```python
from build123d import *

# Parameters (mm, degrees)
SKETCH_2_W          = 110
SKETCH_2_H          = 80
EXTRUDE_1_DEPTH     = 4
EXTRUDE_1_2_DEPTH   = 76
EXTRUDE_2_DEPTH     = 2
CUT_EXTRUDE_1_DEPTH = 90.5
SKETCH_6_R          = 5.5
CUT_EXTRUDE_2_DEPTH = 5
FILLET_1_R          = 10
CUT_EXTRUDE_3_REACH = 61


with BuildPart() as part:
    # Эскиз2 → Extrude 1 (new body)
    with BuildSketch(Plane(origin=(0, 0, 0), x_dir=(1, 0, 0), z_dir=(0, 1, 0))):
        Rectangle(SKETCH_2_W, SKETCH_2_H)
    extrude(amount=EXTRUDE_1_DEPTH)

    # Эскиз3 → Extrude 1 2 (add)
    with BuildSketch(Plane(origin=(0, 4, 0), x_dir=(1, 0, 0), z_dir=(0, 1, 0))):
        with BuildLine():
            Line((-30.5, -15), (-30.5, 14))
            ThreePointArc((-30.5, 14), (-30.207106781, 14.707106781), (-29.5, 15))
            Line((-29.5, 15), (29.5, 15))
            ThreePointArc((29.5, 15), (30.207106781, 14.707106781), (30.5, 14))
            Line((30.5, 14), (30.5, -15))
            Line((30.5, -15), (34.5, -15))
            Line((34.5, -15), (34.5, 14))
            ThreePointArc((34.5, 14), (33.035533906, 17.535533906), (29.5, 19))
            Line((29.5, 19), (-29.5, 19))
            ThreePointArc((-29.5, 19), (-33.035533906, 17.535533906), (-34.5, 14))
            Line((-34.5, 14), (-34.5, -15))
            Line((-34.5, -15), (-30.5, -15))
        make_face()
    extrude(amount=EXTRUDE_1_2_DEPTH)

    # Эскиз4 → Бобышка-Вытянуть2 (add, symmetric)
    with BuildSketch(Plane(origin=(0, 0, 0), x_dir=(0, 0, -1), z_dir=(1, 0, 0))):
        Polygon((19, 31.712812921), (35, 4), (19, 4), align=None)
    extrude(amount=EXTRUDE_2_DEPTH, both=True)

    # Эскиз5 → Вырез-Вытянуть1 (cut, through all)
    with BuildSketch(Plane(origin=(34.5, 0, 0), x_dir=(0, 0, -1), z_dir=(1, 0, 0))):
        with BuildLine():
            Line((5, 68), (5, 56))
            ThreePointArc((5, 56), (0, 51), (-5, 56))
            Line((-5, 56), (-5, 68))
            ThreePointArc((-5, 68), (0, 73), (5, 68))
        make_face()
        with BuildLine():
            Line((5, 28), (5, 16))
            ThreePointArc((5, 16), (0, 11), (-5, 16))
            Line((-5, 16), (-5, 28))
            ThreePointArc((-5, 28), (0, 33), (5, 28))
        make_face()
    extrude(amount=-CUT_EXTRUDE_1_DEPTH, mode=Mode.SUBTRACT)

    # Эскиз6 → Вырез-Вытянуть2 (cut, through all)
    with BuildSketch(Plane(origin=(0, 4, 0), x_dir=(1, 0, 0), z_dir=(0, 1, 0))):
        with Locations(Location((-43, 28, 0), (0, 0, 270))):  # turned: the seam where the file's is
            Circle(SKETCH_6_R)
        with Locations(Location((-43, -28, 0), (0, 0, 270))):  # turned: the seam where the file's is
            Circle(SKETCH_6_R)
        with Locations(Location((43, 28, 0), (0, 0, 270))):  # turned: the seam where the file's is
            Circle(SKETCH_6_R)
        with Locations(Location((43, -28, 0), (0, 0, 270))):  # turned: the seam where the file's is
            Circle(SKETCH_6_R)
    extrude(amount=-CUT_EXTRUDE_2_DEPTH, mode=Mode.SUBTRACT)

    # Скругление1
    fillet_1_edges = [part.edges().sort_by_distance(p)[0] for p in [
        (55, 2, 40),
        (-55, 2, 40),
        (-55, 2, -40),
        (55, 2, -40),
    ]]
    fillet(fillet_1_edges, radius=FILLET_1_R)

    # Эскиз8 → Вырез-Вытянуть3 (cut, up to next)
    with BuildSketch(Plane(origin=(0, 0, -19), x_dir=(-1, 0, 0), z_dir=(0, 0, -1)), mode=Mode.PRIVATE) as cut_extrude_3_sk1:
        with BuildLine():
            Line((-10, 68), (-10, 56))
            ThreePointArc((-10, 56), (-15, 51), (-20, 56))
            Line((-20, 56), (-20, 68))
            ThreePointArc((-20, 68), (-15, 73), (-10, 68))
        make_face()
    cut_extrude_3_tool1 = extrude(cut_extrude_3_sk1.sketch, amount=-CUT_EXTRUDE_3_REACH, mode=Mode.PRIVATE) & part.part
    add(cut_extrude_3_tool1.solids().sort_by_distance((15, 62, -19))[0], mode=Mode.SUBTRACT)
    # Эскиз8 → Вырез-Вытянуть3 (cut, up to next)
    with BuildSketch(Plane(origin=(0, 0, -19), x_dir=(-1, 0, 0), z_dir=(0, 0, -1)), mode=Mode.PRIVATE) as cut_extrude_3_sk2:
        with BuildLine():
            Line((-10, 28), (-10, 16))
            ThreePointArc((-10, 16), (-15, 11), (-20, 16))
            Line((-20, 16), (-20, 28))
            ThreePointArc((-20, 28), (-15, 33), (-10, 28))
        make_face()
    cut_extrude_3_tool2 = extrude(cut_extrude_3_sk2.sketch, amount=-CUT_EXTRUDE_3_REACH, mode=Mode.PRIVATE) & part.part
    add(cut_extrude_3_tool2.solids().sort_by_distance((15, 22, -19))[0], mode=Mode.SUBTRACT)
    # Эскиз8 → Вырез-Вытянуть3 (cut, up to next)
    with BuildSketch(Plane(origin=(0, 0, -19), x_dir=(-1, 0, 0), z_dir=(0, 0, -1)), mode=Mode.PRIVATE) as cut_extrude_3_sk3:
        with BuildLine():
            Line((10, 68), (10, 56))
            ThreePointArc((10, 56), (15, 51), (20, 56))
            Line((20, 56), (20, 68))
            ThreePointArc((20, 68), (15, 73), (10, 68))
        make_face()
    cut_extrude_3_tool3 = extrude(cut_extrude_3_sk3.sketch, amount=-CUT_EXTRUDE_3_REACH, mode=Mode.PRIVATE) & part.part
    add(cut_extrude_3_tool3.solids().sort_by_distance((-15, 62, -19))[0], mode=Mode.SUBTRACT)
    # Эскиз8 → Вырез-Вытянуть3 (cut, up to next)
    with BuildSketch(Plane(origin=(0, 0, -19), x_dir=(-1, 0, 0), z_dir=(0, 0, -1)), mode=Mode.PRIVATE) as cut_extrude_3_sk4:
        with BuildLine():
            Line((10, 28), (10, 16))
            ThreePointArc((10, 16), (15, 11), (20, 16))
            Line((20, 16), (20, 28))
            ThreePointArc((20, 28), (15, 33), (10, 28))
        make_face()
    cut_extrude_3_tool4 = extrude(cut_extrude_3_sk4.sketch, amount=-CUT_EXTRUDE_3_REACH, mode=Mode.PRIVATE) & part.part
    add(cut_extrude_3_tool4.solids().sort_by_distance((-15, 22, -19))[0], mode=Mode.SUBTRACT)


solid = part.part
```
Geometry check sheet. Reference: the model listing, model coordinates, mm. A direction names the side the tool comes from. Round coordinates to 2 decimals unless told otherwise and drop trailing zeros. Order: outer loops, then holes, each group sorted by start corner. A loop starts at its lowest first (then second) coordinate and runs counter-clockwise, first axis right, second up. Notation, with made-up numbers: M -12,-4 L 35,-4 A27 cw 35,32 Z; hole C 47,1.25 d7. An arc over 180 degrees is marked long. Write item = value, one per line.
Q1. Depth check by flat-ended pin: pin 1 Ø10 at (x, z) = (-41, -8) entering from +Y; pin 2 Ø6.5 at (x, z) = (-43, 28) entering from -Y; pin 3 Ø4.5 at (x, y) = (33.5, 59) entering from +Z; pin 4 Ø3 at (x, y) = (34.5, 13) entering from -Z. Enter the tip coordinate at first touch or a pass-through.
Answer block:
pin_1 = 4
pin_2 = through
pin_3 = 15
pin_4 = -17.57
Q2. Section check A-A (x = 43). Enter the section's corners in (y, z).
Answer block:
outline = M 0,-40 L 4,-40 L 4,-33.5 L 0,-33.5 Z; M 0,-22.5 L 4,-22.5 L 4,22.5 L 0,22.5 Z; M 0,33.5 L 4,33.5 L 4,40 L 0,40 Z
Q3. Section check C-C (x = -5.5). Enter the section's corners in (y, z).
Answer block:
outline = M 0,-40 L 4,-40 L 4,-19 L 80,-19 L 80,-15 L 4,-15 L 4,40 L 0,40 Z
Q4. Section check D-D (z = 26). Enter the section's corners in (x, y), plus the area to 3 significant figures.
Answer block:
outline = M -55,0 L -48.12,0 L -48.12,4 L -55,4 Z; M -37.88,0 L 37.88,0 L 37.88,4 L -37.88,4 Z; M 48.12,0 L 55,0 L 55,4 L 48.12,4 Z
area = 358 mm^2
Q5. Scan lines: line 1 (X direction, y = 2.8, z = 28); line 2 (X direction, y = 47, z = -9.5); line 3 (Y direction, x = -25, z = -10). Record each from-to range of solid material in increasing order.
Answer block:
line_1 = -55 to -48.5, -37.5 to 37.5, 48.5 to 55
line_2 = -34.5 to -30.5, 30.5 to 34.5
line_3 = 0 to 4
Q6. Set-up check for faces 1 (the flat face through (30.5, 41, 0)), 2 (the flat face through (-20, 62, -17)), 3 (the cylindrical face through (33.07, 41.47, -17.5)): record each of +Z, -Z, +X, -X, +Y, -Y from which the full face is reachable in a straight line by a thin tool's end or side.
Answer block:
face_1 = +Z, +Y
face_2 = +Z, -Z
face_3 = -Z, +X, +Y
Q7. Release check for a two-part mould opening along Y. For faces 4 (the cylindrical face through (51.99, 2.03, -37.15)), 5 (the flat face through (-10, 22, -17)) record: released by +Y, released by -Y, zero draft, split by the parting line, or undercut.
Answer block:
face_4 = zero draft
face_5 = undercut
Q8. Section check B-B (y = 29.5). Give the number of separate pieces and of enclosed holes in the cut face, plus the area to 3 significant figures.
Answer block:
separate_pieces = 5
enclosed_holes = 0
area = 358 mm^2
